```python
from build123d import *

# Parameters (mm, degrees)
BOSS_EXTRUDE1_DEPTH = 6.35
CUT_EXTRUDE1_START  = -5.715
SKETCH3_R           = 1.27
CUT_EXTRUDE1_DEPTH  = 5.08


with BuildPart() as part:
    # Sketch1 → Boss-Extrude1 (new body)
    with BuildSketch(Plane(origin=(0, 0, 0), x_dir=(1, 0, 0), z_dir=(0, 1, 0))):
        with BuildLine():
            ThreePointArc((-3.272170819, -2.610053381), (-2.267484875, -1.473222208), (-1.905, 0))
            ThreePointArc((-1.905, 0), (-2.267484875, 1.473222208), (-3.272170819, 2.610053381))
            ThreePointArc((-3.272170819, 2.610053381), (-8.255, 0), (-3.272170819, -2.610053381))
        make_face()
        with BuildLine():
            ThreePointArc((-3.272170819, 2.610053381), (-2.267484875, 1.473222208), (-1.905, 0))
            ThreePointArc((-1.905, 0), (-2.267484875, -1.473222208), (-3.272170819, -2.610053381))
            ThreePointArc((-3.272170819, -2.610053381), (0, -1.5875), (3.272170819, -2.610053381))
            ThreePointArc((3.272170819, -2.610053381), (1.905, 0), (3.272170819, 2.610053381))
            ThreePointArc((3.272170819, 2.610053381), (0, 1.5875), (-3.272170819, 2.610053381))
        make_face()
        with BuildLine():
            ThreePointArc((8.255, 0), (6.553222208, 2.812515125), (3.272170819, 2.610053381))
            ThreePointArc((3.272170819, 2.610053381), (1.905, 0), (3.272170819, -2.610053381))
            ThreePointArc((3.272170819, -2.610053381), (6.553222208, -2.812515125), (8.255, 0))
        make_face()
    extrude(amount=BOSS_EXTRUDE1_DEPTH)

    # Sketch3 → Cut-Extrude1 (cut)
    with BuildSketch(Plane(origin=(0, 6.35, 0), x_dir=(1, 0, 0), z_dir=(0, 1, 0)).offset(CUT_EXTRUDE1_START)):
        with BuildLine():
            ThreePointArc((3.272170819, 2.610053381), (0, 1.5875), (-3.272170819, 2.610053381))
            ThreePointArc((-3.272170819, 2.610053381), (-8.255, 0), (-3.272170819, -2.610053381))
            ThreePointArc((-3.272170819, -2.610053381), (0, -1.5875), (3.272170819, -2.610053381))
            ThreePointArc((3.272170819, -2.610053381), (8.255, 0), (3.272170819, 2.610053381))
        make_face()
        with Locations(Location((5.08, 0, 0), (0, 0, 270))):
            Circle(SKETCH3_R, mode=Mode.SUBTRACT)
        with Locations(Location((-5.08, 0, 0), (0, 0, 270))):
            Circle(SKETCH3_R, mode=Mode.SUBTRACT)
    extrude(amount=CUT_EXTRUDE1_DEPTH, mode=Mode.SUBTRACT)


solid = part.part
```
Check sheet for the modelled part. Datum: model origin and axes. Units: mm. A direction names the side the tool comes from. Round coordinates to 2 decimals unless told otherwise and drop trailing zeros. Write each loop counter-clockwise with the first axis right and the second up, starting at its lowest first coordinate (ties: lowest second). Pieces come first, ordered by that corner, then holes. Notation, with made-up numbers: (61.5, 4.25) -> (92.5, 4.25) arc R7 cw to (92.5, 12.25) -> close; hole circle Ø9 at (0.25, 7). An arc over 180 degrees is marked (long way). One line per question, with ' | ' between items. Start each with the question number.
1. Release check for a two-part mould opening along Y. For faces 1 (the face through (0, 0.635, 0)), 2 (the face through (0, 6.35, 0)), 3 (the face through (-3.82, 3.14, -0.17)), 4 (the face through (-8.254, 6.028, -0.097)) record: +Y half, -Y half, draft (parallel to the pull), parting line (faces both ways), or undercut.
2. Sectioned sample at B-B, the plane z = -2.25. Record the cut outline in (x, y) (3 decimals), then the cut area to 3 significant figures.
3. Scan lines: line 1 along Y through (x, z) = (5.5, 2.5) (3 decimals); line 2 along X through (y, z) = (2.5, 0.75); line 3 along X through (y, z) = (3.25, 0.5). Record each from-to range of solid material in increasing order. Write a range as from..to.
4. Depth check by flat-ended pin: pin 1 (1.5 mm diameter, centred on x = -1.5, y = 5.5, fed in from +Z). Enter the tip coordinate at first touch or a pass-through.
5. Sectioned sample at C-C, the plane y = 3.25. Record the cut outline in (x, z), then the cut area to 3 significant figures.
6. Set-up check for faces 5 (the face through (3.84, 3.14, -0.28)), 6 (the face through (-0.049, 6.028, 1.588)): record each of +Z, -Z, +X, -X, +Y, -Y from which the full face is reachable in a straight line by a thin tool's end or side.
7. Sectioned sample at D-D, the plane x = 5.08. Record the cut outline in (y, z) (3 decimals), then the cut area to 3 significant figures.
Taken from the geometry:
1) face 1: undercut | face 2: +Y half | face 3: undercut | face 4: draft
2) outline: (-7.32, 0) -> (-2.679, 0) -> (-2.679, 0.635) -> (-7.32, 0.635) -> close; (-7.32, 5.715) -> (-2.679, 5.715) -> (-2.679, 6.35) -> (-7.32, 6.35) -> close; (2.679, 0) -> (7.32, 0) -> (7.32, 0.635) -> (2.679, 0.635) -> close; (2.679, 5.715) -> (7.32, 5.715) -> (7.32, 6.35) -> (2.679, 6.35) -> close | area: 11.8 mm^2
3) line 1: y = 0..0.635, 5.715..6.35 | line 2: x = -6.1..-4.06, 4.06..6.1 | line 3: x = -6.25..-3.91, 3.91..6.25
4) pin 1: stops at z = 2.03
5) outline: circle Ø2.54 at (-5.08, 0); circle Ø2.54 at (5.08, 0) | area: 10.1 mm^2
6) face 5: none | face 6: +Z, +Y, -Y
7) outline: (0, -3.175) -> (0.635, -3.175) -> (0.635, -1.27) -> (5.715, -1.27) -> (5.715, -3.175) -> (6.35, -3.175) -> (6.35, 3.175) -> (5.715, 3.175) -> (5.715, 1.27) -> (0.635, 1.27) -> (0.635, 3.175) -> (0, 3.175) -> close | area: 21.0 mm^2
